Model file for the job. Use its own axes, mm. A direction names the side the tool comes from. Give positions to 0.01 mm unless a question says otherwise; leave off trailing zeros. Order: outer loops, then holes, each group sorted by start corner. A loop starts at its lowest first (then second) coordinate and runs counter-clockwise, first axis right, second up. Notation, with made-up numbers: (79, 88) - (130, 88) arc R17 ccw to (130, 121) - close; hole circle Ø10 at (-38.75, 83.5). An arc over 180 degrees is marked (long way). Return JSON: item names as keys, results as strings. Group by question number.
from build123d import *

# Parameters (mm, degrees)
SKETCH1_W           = 31
SKETCH1_H           = 55
SKETCH1_R           = 1
SKETCH1_W_2         = 22
SKETCH1_H_2         = 44
BOSS_EXTRUDE1_DEPTH = 3
SKETCH2_W           = 3
SKETCH2_H           = 55
BOSS_EXTRUDE2_DEPTH = 35
SKETCH3_W           = 3
SKETCH3_H           = 53
BOSS_EXTRUDE3_DEPTH = 20
CUT_EXTRUDE1_DEPTH  = 3
SKETCH5_W           = 3
SKETCH5_H           = 38
BOSS_EXTRUDE4_DEPTH = 40
SKETCH6_R           = 1
CUT_EXTRUDE2_DEPTH  = 31
FILLET1_R           = 15


with BuildPart() as part:
    # Sketch1 → Boss-Extrude1 (new body)
    with BuildSketch(Plane.XY):
        with Locations((1.5, 0)):
            Rectangle(SKETCH1_W, SKETCH1_H)
        with Locations((-4.85, -24)):
            Circle(SKETCH1_R, mode=Mode.SUBTRACT)
        with Locations((4.85, -24)):
            Circle(SKETCH1_R, mode=Mode.SUBTRACT)
        with Locations((4.85, 24)):
            Circle(SKETCH1_R, mode=Mode.SUBTRACT)
        with Locations((-4.85, 24)):
            Circle(SKETCH1_R, mode=Mode.SUBTRACT)
        Rectangle(SKETCH1_W_2, SKETCH1_H_2, mode=Mode.SUBTRACT)
    extrude(amount=BOSS_EXTRUDE1_DEPTH)

    # Sketch2 → Boss-Extrude2 (add)
    with BuildSketch(Plane.XY.offset(3)):
        with Locations((15.5, 0)):
            Rectangle(SKETCH2_W, SKETCH2_H)
    extrude(amount=BOSS_EXTRUDE2_DEPTH)

    # Sketch3 → Boss-Extrude3 (add)
    with BuildSketch(Plane(origin=(0, 27.5, 0), x_dir=(1, 0, 0), z_dir=(0, 1, 0))):
        with Locations((15.5, -26.5)):
            Rectangle(SKETCH3_W, SKETCH3_H)
    extrude(amount=BOSS_EXTRUDE3_DEPTH)

    # Sketch4 → Cut-Extrude1 (cut)
    with BuildSketch(Plane.ZY.offset(-14)):
        Polygon((53, 27.5), (38, 27.5), (53, 47.5), align=None)
        Polygon((0, 27.5), (0, 47.5), (15, 47.5), align=None)
    extrude(amount=-CUT_EXTRUDE1_DEPTH, mode=Mode.SUBTRACT)

    # Sketch5 → Boss-Extrude4 (add)
    with BuildSketch(Plane(origin=(0, 47.5, 0), x_dir=(1, 0, 0), z_dir=(0, 1, 0))):
        with Locations((15.5, -34)):
            Rectangle(SKETCH5_W, SKETCH5_H)
    extrude(amount=BOSS_EXTRUDE4_DEPTH)

    # Sketch6 → Cut-Extrude2 (cut)
    with BuildSketch(Plane.ZY.offset(14)):
        with Locations((34, 72)):
            Circle(SKETCH6_R)
        with Locations((34, 75)):
            Circle(SKETCH6_R)
        with Locations((34, 78)):
            Circle(SKETCH6_R)
        with Locations((45.691342951, 71.25)):
            Circle(SKETCH6_R)
        with Locations((43.09326674, 69.75)):
            Circle(SKETCH6_R)
        with Locations((40.495190528, 68.25)):
            Circle(SKETCH6_R)
        with Locations((45.691342951, 57.75)):
            Circle(SKETCH6_R)
        with Locations((43.09326674, 59.25)):
            Circle(SKETCH6_R)
        with Locations((40.495190528, 60.75)):
            Circle(SKETCH6_R)
        with Locations((34, 51)):
            Circle(SKETCH6_R)
        with Locations((34, 54)):
            Circle(SKETCH6_R)
        with Locations((34, 57)):
            Circle(SKETCH6_R)
        with Locations((22.308657049, 57.75)):
            Circle(SKETCH6_R)
        with Locations((24.90673326, 59.25)):
            Circle(SKETCH6_R)
        with Locations((27.504809472, 60.75)):
            Circle(SKETCH6_R)
        with Locations((22.308657049, 71.25)):
            Circle(SKETCH6_R)
        with Locations((24.90673326, 69.75)):
            Circle(SKETCH6_R)
        with Locations((27.504809472, 68.25)):
            Circle(SKETCH6_R)
    extrude(amount=-CUT_EXTRUDE2_DEPTH, mode=Mode.SUBTRACT)

    # Fillet1
    fillet1_edges = [part.edges().sort_by_distance(p)[0] for p in [
        (15.5, 87.5, 53),
        (15.5, 87.5, 15),
    ]]
    fillet(fillet1_edges, radius=FILLET1_R)


solid = part.part
(1) 3-axis set-ups, long thin cutter, end or side, ignore diameter. For faces 4 (the face through (15, -27.5, 12)), 5 (the face through (0, 27.5, 1)), 6 (the face through (11, 0, 1)), 7 (the face through (15, 60, 15)), 8 (the face through (15.48, 57.84, 34.54)): which of +Z, -Z, +X, -X, +Y, -Y reach the whole face in a straight line?
(2) Pull direction X, two halves, no side cores. Call faces 1 (the face through (15.479, 58.426, 44.954)), 2 (the face through (-4.39, 23.11, 1.48)), 3 (the face through (0, 22, 1)): released by +X, released by -X, zero draft, split by the parting line, or undercut.
(3) Slice it at D-D (z = 10.5). Give the cut face in (x, y), and give its area (3 significant figures).
(4) Slice it at C-C (z = 4.5). Give the cut face in (x, y).
(5) Slice it at A-A (x = 9). Give the cut face in (y, z).
(6) Drop flat-ended pins along their axis: pin 1 Ø1.5 at (y, z) = (-9, 37) entering from -X; pin 2 Ø1 at (x, y) = (3.5, 24) entering from +Z; pin 3 Ø1.5 at (x, y) = (15.5, -1) entering from +Z. Give the stop position or say it passes through.
(7) Slice it at B-B (y = 4). Give the cut face in (x, z), and give its area (3 significant figures).
(8) Drill centre lines: L1, parallel to Y at x = -4.85, z = 2.25; L2, parallel to X at y = -14.5, z = 15; L3, parallel to Z at x = -2, y = 23. Where is each one in solid material? Low to high.
Result set:
{
 "1": {"face 4": "+Z, -Z, +X, -X, -Y", "face 5": "+Z, -Z, -X, +Y", "face 6": "+Z, -Z", "face 7": "-Z, +X, -X, +Y", "face 8": "+X, -X"},
 "2": {"face 1": "zero draft", "face 2": "undercut", "face 3": "undercut"},
 "3": {"outline": "(14, -27.5) - (17, -27.5) - (17, 41.5) - (14, 41.5) - close", "area": "207 mm²"},
 "4": {"outline": "(14, -27.5) - (17, -27.5) - (17, 33.5) - (14, 33.5) - close"},
 "5": {"outline": "(-27.5, 0) - (-22, 0) - (-22, 3) - (-27.5, 3) - close; (22, 0) - (27.5, 0) - (27.5, 3) - (22, 3) - close"},
 "6": {"pin 1": "stops at x = 14", "pin 2": "stops at z = 3", "pin 3": "stops at z = 38"},
 "7": {"outline": "(-14, 0) - (-11, 0) - (-11, 3) - (-14, 3) - close; (11, 0) - (17, 0) - (17, 38) - (14, 38) - (14, 3) - (11, 3) - close", "area": "132 mm²"},
 "8": {"L1": "y = -27.5 to -25, -23 to -22, 22 to 23, 25 to 27.5", "L2": "x = 14 to 17", "L3": "z = 0 to 3"}
}
